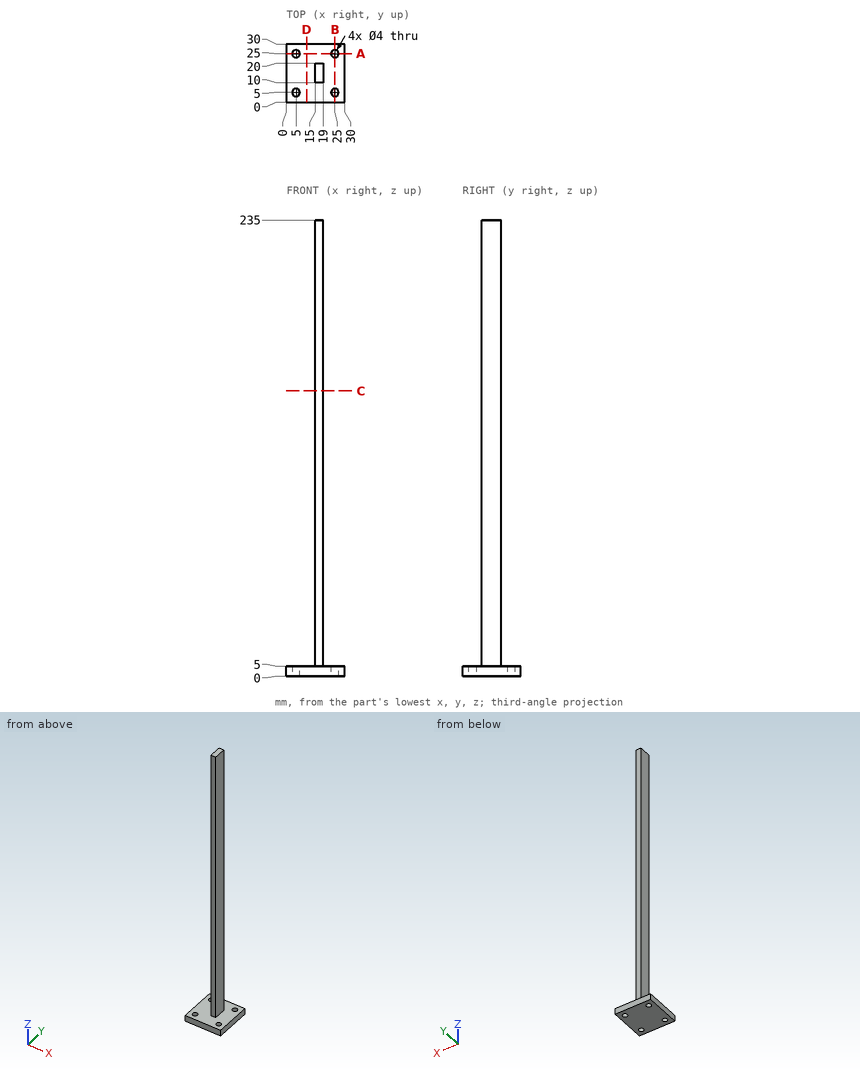
Here's the drawing with two shaded views (mm, measured from the low corner). I have some questions. Give positions to 0.01 mm unless a question says otherwise; leave off trailing zeros. Order: outer loops, then holes, each group sorted by start corner. A loop starts at its lowest first (then second) coordinate and runs counter-clockwise, first axis right, second up. Notation, with made-up numbers: M 67.5,-31 L 116.5,-31 A15 ccw 116.5,-16 Z; hole C -3.5,13 d4. An arc over 180 degrees is marked long. One line per item, written item: value.
1) I want a section at A-A, the plane y = 25. List the corners of the cut face in (x, z) for me.
Answer sheet:
outline: M 0,0 L 3,0 L 3,5 L 0,5 Z; M 7,0 L 23,0 L 23,5 L 7,5 Z; M 27,0 L 30,0 L 30,5 L 27,5 Z
2) I want a section at D-D, the plane x = 10.5. List the corners of the cut face in (y, z) for me.
Answer sheet:
outline: M 0,0 L 30,0 L 30,5 L 0,5 Z
3) I want a section at C-C, the plane z = 147. List the corners of the cut face in (x, y) for me, plus the area to 3 significant figures.
Answer sheet:
outline: M 15,10 L 19,10 L 19,20 L 15,20 Z
area: 40.0 mm^2
4) Please list where these lines run through material, in increasing order: line 1 along Y through (x, z) = (25, 3.2); line 2 along Z through (x, y) = (21.75, 7.5); line 3 along X through (y, z) = (14.25, 92.5).
Answer sheet:
line 1: y = 0 to 3, 7 to 23, 27 to 30
line 2: z = 0 to 5
line 3: x = 15 to 19
5) For P1, Ø1.5, axis at y = 19.5, z = 76, coming from the -X side; P2, Ø2, axis at x = 16, z = 100.5, coming from the -Y side; P3, Ø6, axis at x = 24.5, z = 30, coming from the +Y side; P4, Ø5, axis at x = 12, y = 25, coming from the +Z side, each with a flat end and sliding along its axis, tell me the tip position at first contact or that it passes through.
Answer sheet:
P1: stops at x = 15
P2: stops at y = 10
P3: passes through
P4: stops at z = 5
